Work out the finished part from the listing and answer in its coordinate system (mm). A direction names the side the tool comes from. Give positions to 0.01 mm unless a question says otherwise; leave off trailing zeros. Loops run counter-clockwise (first coordinate to the right, second up) from the corner with the lowest first, then second, coordinate; pieces in that order, holes last. Notation, with made-up numbers: M 88,79.25 L 100,79.25 A20 cw 100,101.25 Z; hole C 4.5,57.5 d3. An arc over 180 degrees is marked long. Answer as a JSON object with one key per item and string values. Group by question number.
```python
from build123d import *

# Parameters (mm, degrees)
SKETCH2_R           = 3.175
BOSS_EXTRUDE1_DEPTH = 12.7
CUT_EXTRUDE1_DEPTH  = 2.286
CHAMFER1_SIZE       = 0.75565


with BuildPart() as part:
    # Sketch1 → Revolve1 (revolve)
    with BuildSketch(Plane(origin=(0, 0, 0), x_dir=(-1, 0, 0), z_dir=(0, 0, -1)), mode=Mode.PRIVATE) as revolve1_sk:
        with BuildLine():
            Line((0, 6.604), (0, 0))
            Line((0, 0), (3.048, 0))
            Line((3.048, 0), (3.048, 2.4384))
            add(Edge.make_bspline(
                [(0.6096, 5.9436), (1.756478304, 5.100704659), (2.65656918, 3.806824025), (3.048, 2.4384)],
                knots=[0, 0, 0, 0, 1, 1, 1, 1], degree=3))
            Line((0.6096, 5.9436), (0.6096, 6.604))
            Line((0.6096, 6.604), (0, 6.604))
        make_face()
    revolve(revolve1_sk.sketch.rotate(Axis((0, 0, 0), (-1, 0, 0)), 270), axis=Axis((0, 0, 0), (-1, 0, 0)))

    # Sketch2 → Boss-Extrude1 (add)
    with BuildSketch(Plane(origin=(0, 0, 0), x_dir=(0, 0, -1), z_dir=(1, 0, 0))):
        Circle(SKETCH2_R)
    extrude(amount=BOSS_EXTRUDE1_DEPTH)

    # Sketch3 → Cut-Extrude1 (cut)
    with BuildSketch(Plane.ZY.offset(3.048)):
        Polygon((0, -2.346351494), (2.032, -1.173175747), (2.032, 1.173175747), (0, 2.346351494), (-2.032, 1.173175747), (-2.032, -1.173175747), align=None)
    extrude(amount=-CUT_EXTRUDE1_DEPTH, mode=Mode.SUBTRACT)

    # Chamfer1
    chamfer1_edges = [part.edges().sort_by_distance(p)[0] for p in [
        (12.7, 0, 3.175),
    ]]
    chamfer(chamfer1_edges, length=CHAMFER1_SIZE)


solid = part.part
```
Item 1: A tool of negligible diameter and unlimited length cuts with its end or side. For faces 1 (the flat face through (-1.92, 1.75, 1.03)), 2 (the cylindrical face through (-0.3, 1.98, 6.3)), from which of +Z, -Z, +X, -X, +Y, -Y can it reach the whole face along a straight path? Write none if from no direction.
Item 2: For a pull along Z with two mould halves and no side action, classify faces 3 (the cylindrical face through (5.89, -3.1, 0.69)), 4 (the flat face through (-1.92, -1.75, -1.03)), 5 (the flat face through (0, -3, -2)) as pulls with the +Z half, pulls with the -Z half, needs draft (parallel to the pull), parting line crosses it, or undercut.
Item 3: Given pin 1 Ø2 at (x, y) = (8.5, -1.5) entering from -Z; pin 2 Ø5 at (x, y) = (7, -1) entering from +Z (3 decimals); pin 3 Ø2 at (x, z) = (10.5, 2) entering from -Y, each flat-ended and moving along its own axis, determine where each tip first touches the part or whether it passes through.
Item 4: Find the intervals of material crossed by probe 1 along X at (y, z) = (-2, -5.75); probe 2 along Z at (x, y) = (-2, 0.75); probe 3 along Z at (x, y) = (-1.5, -1.75), in increasing order. Write a range as [from, to].
Item 5: A cutting plane is placed at A-A (x = 9.5). Determine the outline of the cut face in (y, z) (3 decimals), and give its area (3 significant figures).
The answers:
{
 "1": {"face 1": "-X", "face 2": "+X, -X"},
 "2": {"face 3": "parting line crosses it", "face 4": "undercut", "face 5": "needs draft"},
 "3": {"pin 1": "stops at z = -3.14", "pin 2": "stops at z = 3.175", "pin 3": "stops at y = -3.01"},
 "4": {"probe 1": "x = [-0.61, 0]", "probe 2": "z = [-4.48, -2.03], [2.03, 4.48]", "probe 3": "z = [-4.84, -1.03], [1.03, 4.84]"},
 "5": {"outline": "C 0,0 d6.35", "area": "31.7 mm^2"}
}
